```python
from build123d import *

# Parameters (mm, degrees)
CROQUIS1_R              = 9.5
SALIENTE_EXTRUIR1_DEPTH = 180
SALIENTE_EXTRUIR2_START = -169
CROQUIS2_W              = 5
CROQUIS2_H              = 75
SALIENTE_EXTRUIR2_DEPTH = 150
CROQUIS3_R              = 8.5
CORTAR_EXTRUIR1_DEPTH   = 213.085802537


with BuildPart() as part:
    # Croquis1 → Saliente-Extruir1 (new body)
    with BuildSketch(Plane(origin=(0, 0, 0), x_dir=(0, 0, -1), z_dir=(1, 0, 0))):
        with Locations(Location((0, 0, 0), (0, 0, 180))):
            Circle(CROQUIS1_R)
    extrude(amount=SALIENTE_EXTRUIR1_DEPTH)

    # Croquis2 → Saliente-Extruir2 (add)
    with BuildSketch(Plane.ZY.offset(SALIENTE_EXTRUIR2_START)):
        Polygon((74.139159217, -39.917512185), (71.639159217, -44.247639204), (6.687253933, -6.747639204), (9.187253933, -2.417512185), align=None)
        with Locations((0, 46.66515139)):
            Rectangle(CROQUIS2_W, CROQUIS2_H)
        Polygon((-71.639159217, -44.247639204), (-74.139159217, -39.917512185), (-9.187253933, -2.417512185), (-6.687253933, -6.747639204), align=None)
    extrude(amount=SALIENTE_EXTRUIR2_DEPTH)

    # Croquis3 → Cortar-Extruir1 (cut, through all)
    with BuildSketch(Plane.ZY):
        Circle(CROQUIS3_R)
    extrude(amount=-CORTAR_EXTRUIR1_DEPTH, mode=Mode.SUBTRACT)


solid = part.part
```
Geometry check sheet. Reference: the model listing, model coordinates, mm. A direction names the side the tool comes from. Give positions to 0.01 mm unless a question says otherwise; leave off trailing zeros. Order: outer loops, then holes, each group sorted by start corner. A loop starts at its lowest first (then second) coordinate and runs counter-clockwise, first axis right, second up. Notation, with made-up numbers: (84, -33.5) -> (139, -33.5) arc R32 cw to (139, 1.5) -> close; hole circle Ø2 at (-28.5, 57.5). An arc over 180 degrees is marked (long way). Write each question's results on one line, items separated by ' | '. Start each with the question number.
(1) Sectioned sample at A-A (x = 65.5). Enter the section's corners in (y, z), plus the area to 3 significant figures.
(2) Scan lines: line 1 (Z direction, x = 122.5, y = 0.5); line 2 (Z direction, x = 126.5, y = 63); line 3 (Y direction, x = 62, z = 2). Record each from-to range of solid material in increasing order.
(3) Access from +Z, -Z, +X, -X, +Y, -Y to the whole of each face (thin tool, end or side, straight path). Record for faces 5 (the face through (95, 46, 2.5)), 6 (the face through (169, 47, 0)), 7 (the face through (95.05, -25.76, 39.62)), 8 (the face through (95, 46, -2.5)), 9 (the face through (19, 47, 0)).
(4) Sectioned sample at B-B (z = 0). Enter the section's corners in (x, y), plus the area to 3 significant figures.
(5) Mould release check, pull along Y, two halves, no side actions. Record for faces 1 (the face through (0, 8.4, -2.2)), 2 (the face through (95, 84.165, 0)), 3 (the face through (88.74, 7.167, 4.57)), 4 (the face through (95.05, -25.235, -38.709)): pulls with the +Y half, pulls with the -Y half, needs draft (parallel to the pull), parting line crosses it, or undercut.
(6) Sectioned sample at C-C (y = 0). Enter the section's corners in (x, z).
(7) Gauge pin test, flat ends, axial feed: P1, Ø6, axis at x = 23.5, z = -17, coming from the +Y side; P2, Ø10, axis at x = 118.5, z = -44.5, coming from the +Y side; P3, Ø21, axis at y = -17, z = -48.5, coming from the -X side. Record the tip position at first contact, or that the pin passes through.
(8) Sectioned sample at D-D (y = -17). Enter the section's corners in (x, z).
Answer below:
1) outline: (-44.25, -71.64) -> (-39.92, -74.14) -> (-2.42, -9.19) arc R9.5 ccw to (9.17, -2.5) -> (84.17, -2.5) -> (84.17, 2.5) -> (9.17, 2.5) arc R9.5 ccw to (-2.42, 9.19) -> (-39.92, 74.14) -> (-44.25, 71.64) -> (-6.75, 6.69) arc R9.5 ccw to (-6.75, -6.69) -> close; hole circle Ø17 at (0, 0) | area: 1,180 mm2
2) line 1: -9.49 to -8.49, 8.49 to 9.49 | line 2: -2.5 to 2.5 | line 3: -9.29 to -8.26, 8.26 to 84.17
3) face 5: +Z, +X, -X, +Y | face 6: +Z, -Z, +X, +Y | face 7: +X, -X, -Y | face 8: -Z, +X, -X, +Y | face 9: +Z, -Z, -X, +Y
4) outline: (0, -9.5) -> (180, -9.5) -> (180, -8.5) -> (0, -8.5) -> close; (0, 8.5) -> (180, 8.5) -> (180, 9.5) -> (169, 9.5) -> (169, 84.17) -> (19, 84.17) -> (19, 9.5) -> (0, 9.5) -> close | area: 11,600 mm2
5) face 1: needs draft | face 2: pulls with the +Y half | face 3: undercut | face 4: pulls with the -Y half
6) outline: (0, -9.5) -> (180, -9.5) -> (180, -8.5) -> (0, -8.5) -> close; (0, 8.5) -> (180, 8.5) -> (180, 9.5) -> (0, 9.5) -> close
7) P1: y = -5.2 | P2: y = -19.92 | P3: x = 19
8) outline: (19, -34.44) -> (169, -34.44) -> (169, -24.44) -> (19, -24.44) -> close; (19, 24.44) -> (169, 24.44) -> (169, 34.44) -> (19, 34.44) -> close
